Check sheet for the modelled part. Datum: model origin and axes. Units: mm. Face numbers are marked on the shaded views. Round coordinates to 2 decimals unless told otherwise and drop trailing zeros. Write each loop counter-clockwise with the first axis right and the second up, starting at its lowest first coordinate (ties: lowest second). Pieces come first, ordered by that corner, then holes.
Item 1: Section check C-C, the plane x = -169. Record the cut outline in (y, z).
Item 2: Material ranges on line 1 along X through (y, z) = (5.25, 5.75); line 2 along Y through (x, z) = (-169.25, 8.5); line 3 along Z through (x, y) = (-169, -7.75), recorded low to high.
Item 3: Depth check by flat-ended pin: pin 1 (3 mm diameter, centred on x = -169, y = -5, fed in from +Z). Enter the tip coordinate at first touch or a pass-through.
Item 4: Section check B-B, the plane y = 5. Record the cut outline in (x, z).
Item 5: Release check for a two-part mould opening along Y. For the marked faces 1, 2, 3 and 4 record: pulls with the +Y half, pulls with the -Y half, needs draft (parallel to the pull), parting line crosses it, or undercut.
Item 6: Section check A-A, the plane z = 9. Record the cut outline in (x, y), plus the area to 3 significant figures.
from build123d import *

# Parameters (mm, degrees)
F0_W     = 12
F0_H     = 22
F0_W_2   = 10
F0_H_2   = 20
F1_DEPTH = 5
F2_DEPTH = 25


with BuildPart() as f1:
    # F0 (on Top) → F1 (new body)
    with BuildSketch(Plane.XY):
        with Locations((-170.7817282314, -1.4250520304)):
            Rectangle(F0_W, F0_H)
        with Locations((-170.7817282314, -1.4250520304)):
            Rectangle(F0_W_2, F0_H_2, mode=Mode.SUBTRACT)
        with Locations((-170.7817282314, -1.4250520304)):
            Rectangle(F0_W_2, F0_H_2)
    extrude(amount=F1_DEPTH)

    # F0 (on Top) → F2 (join)
    with BuildSketch(Plane.XY):
        with Locations((-170.7817282314, -1.4250520304)):
            Rectangle(F0_W, F0_H)
        with Locations((-170.7817282314, -1.4250520304)):
            Rectangle(F0_W_2, F0_H_2, mode=Mode.SUBTRACT)
    extrude(amount=F2_DEPTH)


solid = f1.part
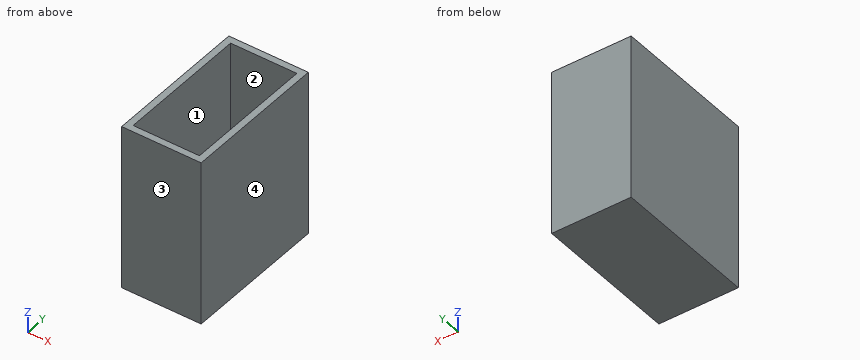
Values found:
1. outline: (-12.43, 0) - (9.57, 0) - (9.57, 25) - (8.57, 25) - (8.57, 5) - (-11.43, 5) - (-11.43, 25) - (-12.43, 25) - close
2. line 1: x = -176.78 to -175.78, -165.78 to -164.78
2. line 2: y = -12.43 to -11.43, 8.57 to 9.57
2. line 3: z = 0 to 5
3. pin 1: stops at z = 5
4. outline: (-176.78, 0) - (-164.78, 0) - (-164.78, 25) - (-165.78, 25) - (-165.78, 5) - (-175.78, 5) - (-175.78, 25) - (-176.78, 25) - close
5. face 1: undercut
5. face 2: undercut
5. face 3: pulls with the -Y half
5. face 4: needs draft
6. outline: (-176.78, -12.43) - (-164.78, -12.43) - (-164.78, 9.57) - (-176.78, 9.57) - close; hole (-175.78, -11.43) - (-165.78, -11.43) - (-165.78, 8.57) - (-175.78, 8.57) - close
6. area: 64.0 mm2
